Input: part model. Units: mm. Frame: model coordinates. Face numbers are marked on the shaded views. A direction names the side the tool comes from. Round coordinates to 2 decimals unless told otherwise and drop trailing zeros. Order: outer loops, then holes, each group sorted by start corner. A loop starts at its lowest first (then second) coordinate and runs counter-clockwise, first axis right, second up. Notation, with made-up numbers: (-32, 69) -> (-1, 69) arc R29 ccw to (-1, 92) -> close; hole circle Ø7 at (60.25, -17.5). An arc over 180 degrees is marked (long way). Use a Markdown table: item, result.
from build123d import *

# Parameters (mm, degrees)
BOSS_EXTRUDE1_DEPTH = 20
FILLET1_R           = 20
FILLET2_R           = 20
SKETCH2_R           = 5
CUT_EXTRUDE2_DEPTH  = 40


with BuildPart() as part:
    # Sketch1 → Boss-Extrude1 (new, symmetric)
    with BuildSketch(Plane(origin=(0, 0, 0), x_dir=(1, 0, 0), z_dir=(0, 1, 0))):
        Polygon((-4.418120101, 15.201487277), (0.581879899, 15.201487277), (0.581879899, -29.798512723), (-24.418120101, -29.798512723), (-24.418120101, -24.798512723), (-4.418120101, -24.798512723), align=None)
    extrude(amount=BOSS_EXTRUDE1_DEPTH, both=True)

    # Fillet1
    fillet1_edges = [part.edges().sort_by_distance(p)[0] for p in [
        (-1.918120101, -20, -15.201487277),
    ]]
    fillet(fillet1_edges, radius=FILLET1_R)

    # Fillet2
    fillet2_edges = [part.edges().sort_by_distance(p)[0] for p in [
        (-1.918120101, 20, -15.201487277),
    ]]
    fillet(fillet2_edges, radius=FILLET2_R - 0.0001)  # a hair under: the kernel refuses the full size

    # Sketch2 → Cut-Extrude2 (cut)
    with BuildSketch(Plane.ZY.offset(4.418120101)):
        with Locations((4.798512723, 0)):
            Circle(SKETCH2_R)
    extrude(amount=-CUT_EXTRUDE2_DEPTH, mode=Mode.SUBTRACT)


solid = part.part
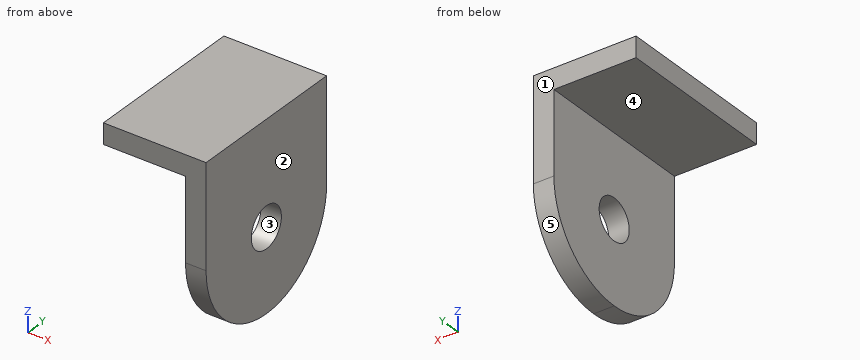
1) Ray query, probe 1 along X at (y, z) = (-13, 0); probe 2 along Z at (x, y) = (-15, 5); probe 3 along Z at (x, y) = (-1.5, -10.5). Return the intervals inside material, ascending.
Answer key:
| item | result |
|---|---|
| probe 1 | x = -4.42 to 0.58 |
| probe 2 | z = 24.8 to 29.8 |
| probe 3 | z = -12.22 to 29.8 |
2) Cut plane D-D on y = -7. Return loops of the section in (x, z), and give its area (3 significant figures).
Answer key:
| item | result |
|---|---|
| outline | (-24.42, 24.8) -> (-4.42, 24.8) -> (-4.42, -13.94) -> (0.58, -13.94) -> (0.58, 29.8) -> (-24.42, 29.8) -> close |
| area | 319 mm^2 |
3) Cut plane A-A on z = 1. Return loops of the section in (x, y).
Answer key:
| item | result |
|---|---|
| outline | (-4.42, -19.64) -> (0.58, -19.64) -> (0.58, -3.25) -> (-4.42, -3.25) -> close; (-4.42, 3.25) -> (0.58, 3.25) -> (0.58, 19.64) -> (-4.42, 19.64) -> close |
4) Cut plane B-B on y = 2.5. Return loops of the section in (x, z), and give its area (3 significant figures).
Answer key:
| item | result |
|---|---|
| outline | (-24.42, 24.8) -> (-4.42, 24.8) -> (-4.42, 9.13) -> (0.58, 9.13) -> (0.58, 29.8) -> (-24.42, 29.8) -> close; (-4.42, -15.04) -> (0.58, -15.04) -> (0.58, 0.47) -> (-4.42, 0.47) -> close |
| area | 281 mm^2 |
5) Contact query for flat-ended pins moving along their axis: P1, Ø13, axis at y = 0, z = 4.8, coming from the -X side; P2, Ø10, axis at x = -16.5, y = 6, coming from the -Z side. Output: stop coordinate, or through.
Answer key:
| item | result |
|---|---|
| P1 | stops at x = -4.42 |
| P2 | stops at z = 24.8 |
6) Cut plane C-C on x = -15. Return loops of the section in (y, z), and give its area (3 significant figures).
Answer key:
| item | result |
|---|---|
| outline | (-20, 24.8) -> (20, 24.8) -> (20, 29.8) -> (-20, 29.8) -> close |
| area | 200 mm^2 |
7) Set-up query: the marked faces 4 and 5. Return all of +Z, -Z, +X, -X, +Y, -Y with unobstructed straight access to the full face (end or side cutting, diameter ignored); none if empty.
Answer key:
| item | result |
|---|---|
| face 4 | -Z, -X, +Y, -Y |
| face 5 | -Z, +X, -X, +Y |
8) Draft query along Y for the marked faces 1, 2 and 3. Return one class per face: released by +Y, released by -Y, zero draft, split by the parting line, or undercut.
Answer key:
| item | result |
|---|---|
| face 1 | released by +Y |
| face 2 | zero draft |
| face 3 | undercut |
